Input: part model. Units: mm. Frame: model coordinates. A direction names the side the tool comes from. Coordinates: 2 decimals unless noted, no trailing zeros. Write each loop counter-clockwise with the first axis right and the second up, starting at its lowest first coordinate (ties: lowest second). Pieces come first, ordered by that corner, then holes. Notation, with made-up numbers: (-29.75, 41.25) - (7.25, 41.25) arc R33 cw to (7.25, 71.25) - close; hole circle Ø6 at (13, -27). An arc over 180 degrees is marked (long way). Use a Markdown table: item, result. Add a question column.
Q1. Section query A-A (z = 1.05). Give the number of separate pieces and of enclosed holes in the cut face, then the cut area to 3 significant figures.
Q2. Mould query, pull axis Y, two halves, no side actions, for faces 4 (the face through (-32.892, 41.432, -0.986)), 5 (the face through (26, -55, 3)), 6 (the face through (24.465, 40.173, 1.479)). Classes: released by +Y, released by -Y, zero draft, split by the parting line, or undercut.
Q3. Pin query (flat end, axial travel): P1, Ø3.5, axis at x = -36.325, y = -36.325, coming from the -Z side; P2, Ø0.9, axis at x = 25, y = -112.5, coming from the +Z side; P3, Ø1.5, axis at x = -27.5, y = 43, coming from the +Z side; P4, Ø1, axis at x = -21, z = -0.5, coming from the +Y side (3 decimals). Return the tip coordinate at first contact, or that it passes through.
Q4. Material intervals for probe 1 along Y at (x, z) = (-27.5, 0.25) (3 decimals); probe 2 along Y at (x, z) = (24.5, 0.85); probe 3 along Z at (x, y) = (5, -117), sorted ascending. Write a range as from..to.
Q5. Set-up query: faces 1 (the face through (-26.801, -55.765, 1.479)), 2 (the face through (-8, -33, -2)), 3 (the face through (-11.28, 34.75, -1.71)). Return all of +Z, -Z, +X, -X, +Y, -Y with unobstructed straight access to the full face (end or side cutting, diameter ignored); none if empty.
Q6. Section query B-B (y = 13). Return the cut outline in (x, z) (3 decimals), then the cut area to 3 significant figures.
from build123d import *

# Parameters (mm, degrees)
SKETCH1_R             = 3.825
SKETCH1_R_2           = 2.525
BOSS_EXTRUDE1_DEPTH   = 3
BOSS_EXTRUDE1_2_DEPTH = 3
BOSS_EXTRUDE1_3_DEPTH = 3
BOSS_EXTRUDE1_4_DEPTH = 3
BOSS_EXTRUDE2_START   = 2
BOSS_EXTRUDE2_DEPTH   = 2
SKETCH4_R             = 1.6
BOSS_EXTRUDE3_DEPTH   = 2
SKETCH6_R             = 2.55
CUT_EXTRUDE1_DEPTH    = 4.2
BOSS_EXTRUDE4_START   = -2
BOSS_EXTRUDE4_DEPTH   = 2
SKETCH10_R            = 2.9
SKETCH10_R_2          = 1.5
BOSS_EXTRUDE5_DEPTH   = 3
CUT_EXTRUDE2_START    = -3.1
SKETCH11_R            = 1.5
CUT_EXTRUDE2_DEPTH    = 3.1
FILLET1_R             = 5
SKETCH12_R            = 1.6
CUT_EXTRUDE3_DEPTH    = 2
CUT_EXTRUDE4_DEPTH    = 1
FILLET2_R             = 1


# Some blends are built 0.0001 mm under size
with BuildPart() as part:
    # Sketch1 → Boss-Extrude1 (new body)
    with BuildSketch(Plane(origin=(0, 0, 0), x_dir=(0, 1, 0), z_dir=(0, 0, 1))):
        with Locations(Location((42.5, 27.5, 0), (0, 0, 270))):
            Circle(SKETCH1_R)
        with Locations(Location((42.5, 27.5, 0), (0, 0, 270))):
            Circle(SKETCH1_R_2, mode=Mode.SUBTRACT)
    extrude(amount=BOSS_EXTRUDE1_DEPTH)



with BuildPart() as body_2:
    # Sketch1 → Boss-Extrude1 2 (new body)
    with BuildSketch(Plane(origin=(0, 0, 0), x_dir=(0, 1, 0), z_dir=(0, 0, 1))):
        with Locations(Location((-42.5, 27.5, 0), (0, 0, 270))):
            Circle(SKETCH1_R)
        with Locations(Location((-42.5, 27.5, 0), (0, 0, 270))):
            Circle(SKETCH1_R_2, mode=Mode.SUBTRACT)
    extrude(amount=BOSS_EXTRUDE1_2_DEPTH)


with BuildPart() as body_3:
    # Sketch1 → Boss-Extrude1 3 (new body)
    with BuildSketch(Plane(origin=(0, 0, 0), x_dir=(0, 1, 0), z_dir=(0, 0, 1))):
        with Locations(Location((-42.5, -27.5, 0), (0, 0, 270))):
            Circle(SKETCH1_R)
        with Locations(Location((-42.5, -27.5, 0), (0, 0, 270))):
            Circle(SKETCH1_R_2, mode=Mode.SUBTRACT)
    extrude(amount=BOSS_EXTRUDE1_3_DEPTH)


with BuildPart() as body_4:
    # Sketch1 → Boss-Extrude1 4 (new body)
    with BuildSketch(Plane(origin=(0, 0, 0), x_dir=(0, 1, 0), z_dir=(0, 0, 1))):
        with Locations(Location((42.5, -27.5, 0), (0, 0, 270))):
            Circle(SKETCH1_R)
        with Locations(Location((42.5, -27.5, 0), (0, 0, 270))):
            Circle(SKETCH1_R_2, mode=Mode.SUBTRACT)
    extrude(amount=BOSS_EXTRUDE1_4_DEPTH)


with BuildPart() as part_1:
    add(part.part)

    add(body_2.part)  # Boss-Extrude2 merges body 2

    add(body_3.part)  # Boss-Extrude2 merges body 3

    add(body_4.part)  # Boss-Extrude2 merges body 4
    # Sketch3 → Boss-Extrude2 (add)
    with BuildSketch(Plane(origin=(0, 0, 0), x_dir=(1, 0, 0), z_dir=(0, 0, -1)).offset(BOSS_EXTRUDE2_START)):
        with BuildLine():
            Line((-31.325, -42.5), (-31.325, 42.5))
            ThreePointArc((-31.325, 42.5), (-30.204683438, 45.204683438), (-27.5, 46.325))
            Line((-27.5, 46.325), (27.5, 46.325))
            ThreePointArc((27.5, 46.325), (30.204683438, 45.204683438), (31.325, 42.5))
            Line((31.325, 42.5), (31.325, -42.5))
            ThreePointArc((31.325, -42.5), (30.204683438, -45.204683438), (27.5, -46.325))
            Line((27.5, -46.325), (-27.5, -46.325))
            ThreePointArc((-27.5, -46.325), (-30.204683438, -45.204683438), (-31.325, -42.5))
        make_face()
    extrude(amount=-BOSS_EXTRUDE2_DEPTH)

    # Sketch4 → Boss-Extrude3 (add)
    # profile 1 of 2: a face of its own
    with BuildSketch(Plane.XY):
        Polygon((-27.5, -46.325), (-45.325, -46.325), (-45.325, 40.5), (-31.325, 40.5), (-31.325, -42.5), align=None)
        with Locations((-36.325, 20.5)):
            Circle(SKETCH4_R, mode=Mode.SUBTRACT)
        with Locations((-36.325, -36.325)):
            Circle(SKETCH4_R, mode=Mode.SUBTRACT)
    # profile 2 of 2: a face of its own
    with BuildSketch(Plane.XY):
        Polygon((31.325, 42.5), (31.325, 68.325), (-21.5, 68.325), (-21.5, 46.325), (27.5, 46.325), align=None)
        with Locations((21.325, 59.325)):
            Circle(SKETCH4_R, mode=Mode.SUBTRACT)
        with Locations((-1.5, 59.325)):
            Circle(SKETCH4_R, mode=Mode.SUBTRACT)
    extrude(amount=-BOSS_EXTRUDE3_DEPTH)

    # Sketch6 → Cut-Extrude1 (cut)
    with BuildSketch(Plane.XY.offset(3)):
        with Locations((-27.5, 42.5)):
            Circle(SKETCH6_R)
        with Locations((27.5, 42.5)):
            Circle(SKETCH6_R)
        with Locations((27.5, -42.5)):
            Circle(SKETCH6_R)
        with Locations((-27.5, -42.5)):
            Circle(SKETCH6_R)
    extrude(amount=-CUT_EXTRUDE1_DEPTH, mode=Mode.SUBTRACT)

    # Sketch9 → Boss-Extrude4 (add)
    with BuildSketch(Plane.XY.offset(BOSS_EXTRUDE4_START)):
        with BuildLine():
            Line((-45.325, -46.325), (27.5, -46.325))
            ThreePointArc((27.5, -46.325), (30.204683438, -45.204683438), (31.325, -42.5))
            Line((31.325, -42.5), (31.325, -137))
            Line((31.325, -137), (-45.325, -137))
            Line((-45.325, -137), (-45.325, -46.325))
        make_face()
    extrude(amount=BOSS_EXTRUDE4_DEPTH)

    # Sketch10 → Boss-Extrude5 (add)
    # profile 1 of 4: a face of its own
    with BuildSketch(Plane.XY):
        with Locations((-24.5, -112)):
            Circle(SKETCH10_R)
        with Locations((-24.5, -112)):
            Circle(SKETCH10_R_2, mode=Mode.SUBTRACT)
    # profile 2 of 4: a face of its own
    with BuildSketch(Plane.XY):
        with Locations((-24.5, -54)):
            Circle(SKETCH10_R)
        with Locations((-24.5, -54)):
            Circle(SKETCH10_R_2, mode=Mode.SUBTRACT)
    # profile 3 of 4: a face of its own
    with BuildSketch(Plane.XY):
        with Locations((24.5, -54)):
            Circle(SKETCH10_R)
        with Locations((24.5, -54)):
            Circle(SKETCH10_R_2, mode=Mode.SUBTRACT)
    # profile 4 of 4: a face of its own
    with BuildSketch(Plane.XY):
        with Locations((24.5, -112)):
            Circle(SKETCH10_R)
        with Locations((24.5, -112)):
            Circle(SKETCH10_R_2, mode=Mode.SUBTRACT)
    extrude(amount=BOSS_EXTRUDE5_DEPTH)

    # Sketch11 → Cut-Extrude2 (cut)
    with BuildSketch(Plane.XY.offset(3).offset(CUT_EXTRUDE2_START)):
        with Locations((-24.5, -112)):
            Circle(SKETCH11_R)
        with Locations((24.5, -112)):
            Circle(SKETCH11_R)
        with Locations((24.5, -54)):
            Circle(SKETCH11_R)
        with Locations((-24.5, -54)):
            Circle(SKETCH11_R)
    extrude(amount=CUT_EXTRUDE2_DEPTH, mode=Mode.SUBTRACT)

    # Fillet1
    # the kernel refuses this fillet: 5 mm, written as the material it adds along each edge
    with BuildSketch(Plane(origin=(-21.5, 46.325, 0), x_dir=(-1, 0, 0), z_dir=(0, 0, -1))) as fillet1_piece_1:
        with BuildLine():
            CenterArc((FILLET1_R, FILLET1_R), FILLET1_R, 180, 90)
            Line((0, FILLET1_R), (0, 0))
            Line((0, 0), (FILLET1_R, 0))
        make_face()
    extrude(amount=2)
    with BuildSketch(Plane(origin=(-31.325, 40.5, 0), x_dir=(-1, 0, 0), z_dir=(0, 0, -1))) as fillet1_piece_2:
        with BuildLine():
            CenterArc((4.474435222, 5), FILLET1_R, 199.873422245, 70.126577755)
            Line((-0.227794366, 3.300283286), (-0.698017324, 3.130311615))
            ThreePointArc((-0.698017324, 3.130311615), (-0.5, 2), (-0.5, 0))
            Line((-0.5, 0), (0, -0.5))
            Line((0, -0.5), (4.474435222, -0.5))
            Line((4.474435222, -0.5), (4.474435222, 0))
        make_face()
    extrude(amount=2)
    # the kernel refuses this fillet: 5 mm, written as the material it takes off along each edge
    with BuildSketch(Plane(origin=(-45.325, 40.5, 12.5), x_dir=(0, -1, 0), z_dir=(0, 0, -1)), Plane(origin=(-21.5, 68.325, 12.5), x_dir=(0, -1, 0), z_dir=(0, 0, -1)), Plane(origin=(31.325, 68.325, 12.5), x_dir=(-1, 0, 0), z_dir=(0, 0, -1))) as fillet1_2_piece_1:
        with BuildLine():
            CenterArc((FILLET1_R, -FILLET1_R), FILLET1_R, 90, 90)
            Line((0, -FILLET1_R), (0, 0))
            Line((0, 0), (FILLET1_R, 0))
        make_face()
    extrude(amount=27, mode=Mode.SUBTRACT)
    with BuildSketch(Plane(origin=(-45.325, -137, -14.5), x_dir=(1, 0, 0), z_dir=(0, 0, 1)), Plane(origin=(31.325, -137, -14.5), x_dir=(0, 1, 0), z_dir=(0, 0, 1))) as fillet1_2_piece_2:
        with BuildLine():
            CenterArc((FILLET1_R, FILLET1_R), FILLET1_R, 180, 90)
            Line((0, FILLET1_R), (0, 0))
            Line((0, 0), (FILLET1_R, 0))
        make_face()
    extrude(amount=27, mode=Mode.SUBTRACT)

    # Sketch12 → Cut-Extrude3 (cut)
    with BuildSketch(Plane.XY):
        with Locations((-36.325, -127)):
            Circle(SKETCH12_R)
        with Locations((-36.325, -82.7952358)):
            Circle(SKETCH12_R)
    extrude(amount=-CUT_EXTRUDE3_DEPTH, mode=Mode.SUBTRACT)

    # Sketch14 → Cut-Extrude4 (cut)
    with BuildSketch(Plane.YX.offset(2)):
        with BuildLine():
            Line((19.725, -26.725), (49.725, 3.275))
            Line((49.725, 3.275), (49.725, -24.741163405))
            Line((49.725, -24.741163405), (45.149423643, -24.741163405))
            ThreePointArc((45.149423643, -24.741163405), (41.366713749, -23.846742923), (38.75433584, -26.725))
            Line((38.75433584, -26.725), (19.725, -26.725))
        make_face()
    extrude(amount=-CUT_EXTRUDE4_DEPTH, mode=Mode.SUBTRACT)

    # Fillet2
    fillet2_edges = [part_1.edges().sort_by_distance(p)[0] for p in [
        (-24.741163405, 45.896993144, -2),
        (-23.846742923, 41.366713749, -2),
        (-26.725, 29.23966792, -2),
        (-9.243956144, 49.725, -2),
        (-11.725, 34.725, -2),
    ]]
    fillet(fillet2_edges, radius=FILLET2_R - 0.0001)  # a hair under: the kernel refuses the full size


solid = part_1.part
Values follow:
| question | item | result |
|---|---|---|
| 1 | separate pieces | 8 |
| 1 | enclosed holes | 8 |
| 1 | area | 180 mm2 |
| 2 | face 4 | released by +Y |
| 2 | face 5 | zero draft |
| 2 | face 6 | undercut |
| 3 | P1 | z = -2 |
| 3 | P2 | z = -0.1 |
| 3 | P3 | z = -1.2 |
| 3 | P4 | y = 66.325 |
| 4 | probe 1 | -46.325..-45.05, -39.95..-38.675, 38.675..39.95, 45.05..46.325 |
| 4 | probe 2 | -114.9..-113.5, -110.5..-109.1, -56.9..-55.5, -52.5..-51.1, -44.87..-40.13, 40.13..44.87 |
| 4 | probe 3 | -2..0 |
| 5 | face 1 | +Z |
| 5 | face 2 | -Z, +X, -X, +Y, -Y |
| 5 | face 3 | -Z |
| 6 | outline | (-45.325, -2) - (31.325, -2) - (31.325, 0) - (-45.325, 0) - close |
| 6 | area | 153 mm2 |
